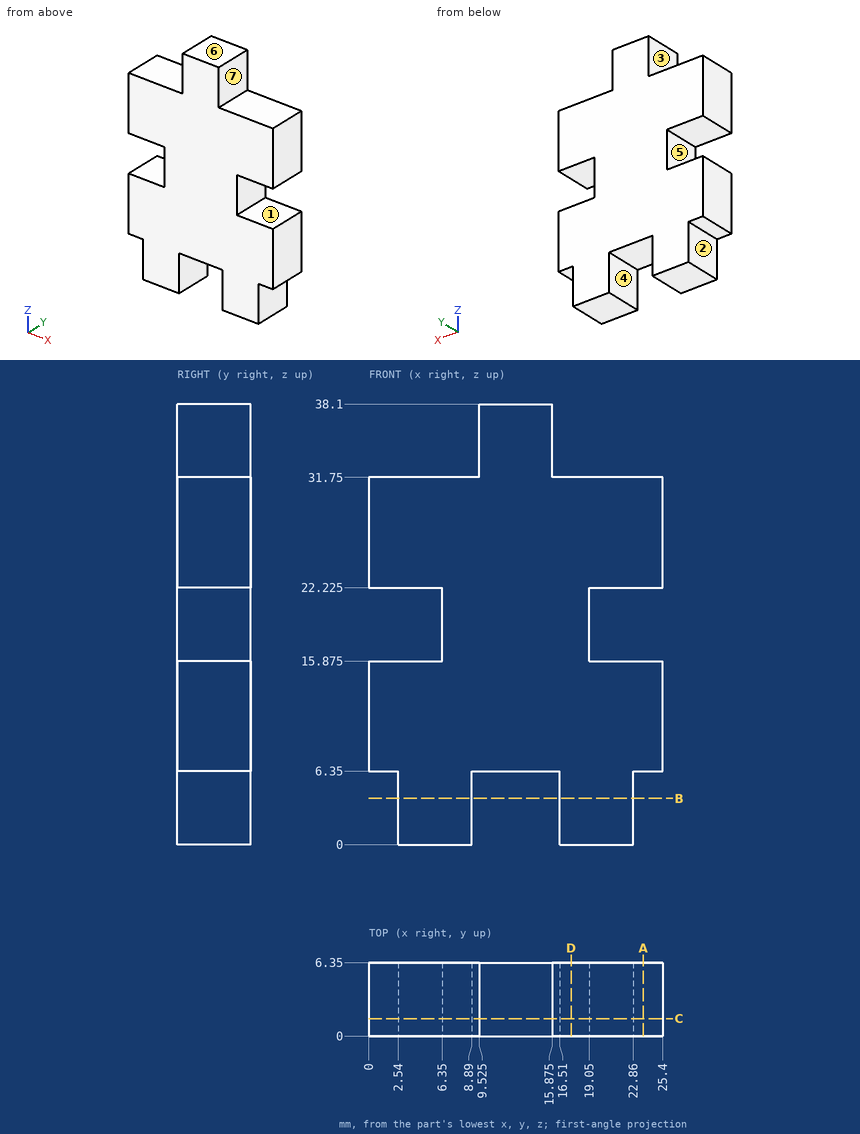
Design review of the part shown in the three views and the two pictorial views. Dimensions are in mm from the part's minimum x, y and z. A direction names the side the tool comes from. Round coordinates to 2 decimals unless told otherwise and drop trailing zeros. Order: outer loops, then holes, each group sorted by start corner. A loop starts at its lowest first (then second) coordinate and runs counter-clockwise, first axis right, second up.
Item 1: Add section C-C, the plane y = 1.5. State the section outline as (x, z) points (3 decimals).
Working result:
outline: (0, 6.35) - (2.54, 6.35) - (2.54, 0) - (8.89, 0) - (8.89, 6.35) - (16.51, 6.35) - (16.51, 0) - (22.86, 0) - (22.86, 6.35) - (25.4, 6.35) - (25.4, 15.875) - (19.05, 15.875) - (19.05, 22.225) - (25.4, 22.225) - (25.4, 31.75) - (15.875, 31.75) - (15.875, 38.1) - (9.525, 38.1) - (9.525, 31.75) - (0, 31.75) - (0, 22.225) - (6.35, 22.225) - (6.35, 15.875) - (0, 15.875) - close
Item 2: Add section D-D, the plane x = 17.5. State the section outline as (y, z) points, and give its area (3 significant figures).
Working result:
outline: (0, 0) - (6.35, 0) - (6.35, 31.75) - (0, 31.75) - close
area: 202 mm2
Item 3: Machinability: for the marked faces 1, 2, 3 and 4, which of the approach directions +Z, -Z, +X, -X, +Y, -Y give a long, thin tool a straight path to every point of the face, cutting with its end or side? Answer none if there is none.
Working result:
face 1: +X, +Y, -Y
face 2: -Z, -X, +Y, -Y
face 3: +Z, -X, +Y, -Y
face 4: -Z, +Y, -Y
Item 4: Add section A-A, the plane x = 23.75. State the section outline as (y, z) points (3 decimals).
Working result:
outline: (0, 6.35) - (6.35, 6.35) - (6.35, 15.875) - (0, 15.875) - close; (0, 22.225) - (6.35, 22.225) - (6.35, 31.75) - (0, 31.75) - close
Item 5: Draft analysis for pull direction Z (two halves, no side actions). For the marked faces 5, 6 and 7, state which applies: released by +Z, released by -Z, zero draft, split by the parting line, or undercut.
Working result:
face 5: undercut
face 6: released by +Z
face 7: zero draft
Item 6: Add section B-B, the plane z = 4. State the section outline as (x, y) points, and give its area (3 significant figures).
Working result:
outline: (2.54, 0) - (8.89, 0) - (8.89, 6.35) - (2.54, 6.35) - close; (16.51, 0) - (22.86, 0) - (22.86, 6.35) - (16.51, 6.35) - close
area: 80.6 mm2
Item 7: For pin 1 (3 mm diameter, centred on x = 22.5, y = 2, fed in from -Z); pin 2 (3 mm diameter, centred on x = 20, y = 3, fed in from +Z); pin 3 (0.8 mm diameter, centred on x = 23.5, y = 2, fed in from -Z); pin 4 (3 mm diameter, centred on y = 2, z = 20, fed in from +X), all flat-tipped, find the tip position at first contact; note any pin that passes through.
Working result:
pin 1: stops at z = 0
pin 2: stops at z = 31.75
pin 3: stops at z = 6.35
pin 4: stops at x = 19.05
Item 8: To check wall thickness, follow probe 1 along Z at (x, y) = (22.5, 4.75) (3 decimals); probe 2 along X at (y, z) = (2.5, 4); probe 3 along Z at (x, y) = (1.75, 5.5) (3 decimals). State the ranges of each line that lie inside material, in increasing order.
Working result:
probe 1: z = 0 to 15.875, 22.225 to 31.75
probe 2: x = 2.54 to 8.89, 16.51 to 22.86
probe 3: z = 6.35 to 15.875, 22.225 to 31.75
